from build123d import *

# Parameters (mm, degrees)
SKETCH1_R           = 2
BOSS_EXTRUDE1_DEPTH = 3


with BuildPart() as part:
    # Sketch1 → Boss-Extrude1 (new body)
    with BuildSketch(Plane(origin=(0, 0, 0), x_dir=(1, 0, 0), z_dir=(0, 1, 0))):
        Polygon((-117.708234781, 46.18565323), (-117.708234781, 37.539058804), (-104.708234781, 37.539058804), (-104.708234781, -32.460941196), (-117.708234781, -32.460941196), (-117.708234781, -41.961747622), (-102.708234781, -57.460941196), (-32.708234781, -57.460941196), (-17.708234781, -41.961747622), (-17.708234781, -32.460941196), (-30.708234781, -32.460941196), (-30.708234781, 37.539058804), (-17.708234781, 37.539058804), (-17.708234781, 48.362937983), (-32.482765457, 62.539058804), (-102.482765457, 62.539058804), (-117.673238758, 46.131294908), align=None)
        with Locations((-96.708234781, 16.539058804)):
            Circle(SKETCH1_R, mode=Mode.SUBTRACT)
        with Locations((-96.708234781, -11.460941196)):
            Circle(SKETCH1_R, mode=Mode.SUBTRACT)
        with Locations((-102.708234781, -48.800687158)):
            Circle(SKETCH1_R, mode=Mode.SUBTRACT)
        with Locations((-67.708234781, -48.800687158)):
            Circle(SKETCH1_R, mode=Mode.SUBTRACT)
        with Locations((-102.708234781, 53.878804766)):
            Circle(SKETCH1_R, mode=Mode.SUBTRACT)
        with Locations((-67.708234781, 53.878804766)):
            Circle(SKETCH1_R, mode=Mode.SUBTRACT)
        with Locations((-32.708234781, 53.878804766)):
            Circle(SKETCH1_R, mode=Mode.SUBTRACT)
        with Locations((-32.708234781, -48.800687158)):
            Circle(SKETCH1_R, mode=Mode.SUBTRACT)
        with Locations((-38.708234781, -11.460941196)):
            Circle(SKETCH1_R, mode=Mode.SUBTRACT)
        with Locations((-38.708234781, 16.539058804)):
            Circle(SKETCH1_R, mode=Mode.SUBTRACT)
        with Locations((-52.771353365, 2.539058804)):
            Circle(SKETCH1_R, mode=Mode.SUBTRACT)
        with Locations((-82.645116197, 2.539058804)):
            Circle(SKETCH1_R, mode=Mode.SUBTRACT)
        with BuildLine():
            Line((-79.583025643, 48.362937983), (-79.583025643, 23.355939616))
            ThreePointArc((-79.583025643, 23.355939616), (-81.595082983, 21.343882276), (-83.607140323, 23.355939616))
            Line((-83.607140323, 23.355939616), (-83.607140323, 48.362937983))
            ThreePointArc((-83.607140323, 48.362937983), (-81.595082983, 50.374995323), (-79.583025643, 48.362937983))
        make_face(mode=Mode.SUBTRACT)
        with BuildLine():
            Line((-71.954133984, 48.07550122), (-71.954133984, 23.068502853))
            ThreePointArc((-71.954133984, 23.068502853), (-73.966191324, 21.056445514), (-75.978248664, 23.068502853))
            Line((-75.978248664, 23.068502853), (-75.978248664, 48.07550122))
            ThreePointArc((-75.978248664, 48.07550122), (-73.966191324, 50.08755856), (-71.954133984, 48.07550122))
        make_face(mode=Mode.SUBTRACT)
        with BuildLine():
            Line((-73.966191324, 14.281397024), (-91.218060864, 14.281397024))
            ThreePointArc((-91.218060864, 14.281397024), (-93.048616644, 16.111952804), (-91.218060864, 17.942508584))
            Line((-91.218060864, 17.942508584), (-73.966191324, 17.942508584))
            ThreePointArc((-73.966191324, 17.942508584), (-72.135635543, 16.111952804), (-73.966191324, 14.281397024))
        make_face(mode=Mode.SUBTRACT)
        with BuildLine():
            Line((-96.834895183, 48.362937983), (-96.834895183, 23.355939616))
            ThreePointArc((-96.834895183, 23.355939616), (-98.846952522, 21.343882276), (-100.859009862, 23.355939616))
            Line((-100.859009862, 23.355939616), (-100.859009862, 48.362937983))
            ThreePointArc((-100.859009862, 48.362937983), (-98.846952522, 50.374995323), (-96.834895183, 48.362937983))
        make_face(mode=Mode.SUBTRACT)
        with BuildLine():
            Line((-89.206003524, 48.07550122), (-89.206003524, 23.068502853))
            ThreePointArc((-89.206003524, 23.068502853), (-91.218060864, 21.056445514), (-93.230118203, 23.068502853))
            Line((-93.230118203, 23.068502853), (-93.230118203, 48.07550122))
            ThreePointArc((-93.230118203, 48.07550122), (-91.218060864, 50.08755856), (-89.206003524, 48.07550122))
        make_face(mode=Mode.SUBTRACT)
        with BuildLine():
            Line((-55.727463713, 48.362937983), (-55.727463713, 23.355939616))
            ThreePointArc((-55.727463713, 23.355939616), (-53.715406373, 21.343882276), (-51.703349033, 23.355939616))
            Line((-51.703349033, 23.355939616), (-51.703349033, 48.362937983))
            ThreePointArc((-51.703349033, 48.362937983), (-53.715406373, 50.374995323), (-55.727463713, 48.362937983))
        make_face(mode=Mode.SUBTRACT)
        with BuildLine():
            Line((-63.356355372, 48.07550122), (-63.356355372, 23.068502853))
            ThreePointArc((-63.356355372, 23.068502853), (-61.344298032, 21.056445514), (-59.332240692, 23.068502853))
            Line((-59.332240692, 23.068502853), (-59.332240692, 48.07550122))
            ThreePointArc((-59.332240692, 48.07550122), (-61.344298032, 50.08755856), (-63.356355372, 48.07550122))
        make_face(mode=Mode.SUBTRACT)
        with BuildLine():
            Line((-38.475594173, 48.362937983), (-38.475594173, 23.355939616))
            ThreePointArc((-38.475594173, 23.355939616), (-36.463536833, 21.343882276), (-34.451479493, 23.355939616))
            Line((-34.451479493, 23.355939616), (-34.451479493, 48.362937983))
            ThreePointArc((-34.451479493, 48.362937983), (-36.463536833, 50.374995323), (-38.475594173, 48.362937983))
        make_face(mode=Mode.SUBTRACT)
        with BuildLine():
            Line((-46.104485832, 48.07550122), (-46.104485832, 23.068502853))
            ThreePointArc((-46.104485832, 23.068502853), (-44.092428492, 21.056445514), (-42.080371152, 23.068502853))
            Line((-42.080371152, 23.068502853), (-42.080371152, 48.07550122))
            ThreePointArc((-42.080371152, 48.07550122), (-44.092428492, 50.08755856), (-46.104485832, 48.07550122))
        make_face(mode=Mode.SUBTRACT)
        with BuildLine():
            Line((-79.583025643, -44.139032376), (-79.583025643, -19.132034009))
            ThreePointArc((-79.583025643, -19.132034009), (-81.595082983, -17.119976669), (-83.607140323, -19.132034009))
            Line((-83.607140323, -19.132034009), (-83.607140323, -44.139032376))
            ThreePointArc((-83.607140323, -44.139032376), (-81.595082983, -46.151089715), (-79.583025643, -44.139032376))
        make_face(mode=Mode.SUBTRACT)
        with BuildLine():
            Line((-71.954133984, -43.851595613), (-71.954133984, -18.844597246))
            ThreePointArc((-71.954133984, -18.844597246), (-73.966191324, -16.832539906), (-75.978248664, -18.844597246))
            Line((-75.978248664, -18.844597246), (-75.978248664, -43.851595613))
            ThreePointArc((-75.978248664, -43.851595613), (-73.966191324, -45.863652953), (-71.954133984, -43.851595613))
        make_face(mode=Mode.SUBTRACT)
        with BuildLine():
            Line((-96.834895183, -44.139032376), (-96.834895183, -19.132034009))
            ThreePointArc((-96.834895183, -19.132034009), (-98.846952522, -17.119976669), (-100.859009862, -19.132034009))
            Line((-100.859009862, -19.132034009), (-100.859009862, -44.139032376))
            ThreePointArc((-100.859009862, -44.139032376), (-98.846952522, -46.151089715), (-96.834895183, -44.139032376))
        make_face(mode=Mode.SUBTRACT)
        with BuildLine():
            Line((-89.206003524, -43.851595613), (-89.206003524, -18.844597246))
            ThreePointArc((-89.206003524, -18.844597246), (-91.218060864, -16.832539906), (-93.230118203, -18.844597246))
            Line((-93.230118203, -18.844597246), (-93.230118203, -43.851595613))
            ThreePointArc((-93.230118203, -43.851595613), (-91.218060864, -45.863652953), (-89.206003524, -43.851595613))
        make_face(mode=Mode.SUBTRACT)
        with BuildLine():
            Line((-55.727463713, -44.139032376), (-55.727463713, -19.132034009))
            ThreePointArc((-55.727463713, -19.132034009), (-53.715406373, -17.119976669), (-51.703349033, -19.132034009))
            Line((-51.703349033, -19.132034009), (-51.703349033, -44.139032376))
            ThreePointArc((-51.703349033, -44.139032376), (-53.715406373, -46.151089715), (-55.727463713, -44.139032376))
        make_face(mode=Mode.SUBTRACT)
        with BuildLine():
            Line((-63.356355372, -43.851595613), (-63.356355372, -18.844597246))
            ThreePointArc((-63.356355372, -18.844597246), (-61.344298032, -16.832539906), (-59.332240692, -18.844597246))
            Line((-59.332240692, -18.844597246), (-59.332240692, -43.851595613))
            ThreePointArc((-59.332240692, -43.851595613), (-61.344298032, -45.863652953), (-63.356355372, -43.851595613))
        make_face(mode=Mode.SUBTRACT)
        with BuildLine():
            Line((-38.475594173, -44.139032376), (-38.475594173, -19.132034009))
            ThreePointArc((-38.475594173, -19.132034009), (-36.463536833, -17.119976669), (-34.451479493, -19.132034009))
            Line((-34.451479493, -19.132034009), (-34.451479493, -44.139032376))
            ThreePointArc((-34.451479493, -44.139032376), (-36.463536833, -46.151089715), (-38.475594173, -44.139032376))
        make_face(mode=Mode.SUBTRACT)
        with BuildLine():
            Line((-46.104485832, -43.851595613), (-46.104485832, -18.844597246))
            ThreePointArc((-46.104485832, -18.844597246), (-44.092428492, -16.832539906), (-42.080371152, -18.844597246))
            Line((-42.080371152, -18.844597246), (-42.080371152, -43.851595613))
            ThreePointArc((-42.080371152, -43.851595613), (-44.092428492, -45.863652953), (-46.104485832, -43.851595613))
        make_face(mode=Mode.SUBTRACT)
        with BuildLine():
            Line((-73.966191324, 7.984384289), (-91.218060864, 7.984384289))
            ThreePointArc((-91.218060864, 7.984384289), (-92.918765354, 9.685088779), (-91.218060864, 11.385793269))
            Line((-91.218060864, 11.385793269), (-73.966191324, 11.385793269))
            ThreePointArc((-73.966191324, 11.385793269), (-72.265486834, 9.685088779), (-73.966191324, 7.984384289))
        make_face(mode=Mode.SUBTRACT)
        with BuildLine():
            Line((-61.344298032, 14.281397024), (-44.092428492, 14.281397024))
            ThreePointArc((-44.092428492, 14.281397024), (-42.261872712, 16.111952804), (-44.092428492, 17.942508584))
            Line((-44.092428492, 17.942508584), (-61.344298032, 17.942508584))
            ThreePointArc((-61.344298032, 17.942508584), (-63.174853812, 16.111952804), (-61.344298032, 14.281397024))
        make_face(mode=Mode.SUBTRACT)
        with BuildLine():
            Line((-61.344298032, 7.984384289), (-44.092428492, 7.984384289))
            ThreePointArc((-44.092428492, 7.984384289), (-42.391724002, 9.685088779), (-44.092428492, 11.385793269))
            Line((-44.092428492, 11.385793269), (-61.344298032, 11.385793269))
            ThreePointArc((-61.344298032, 11.385793269), (-63.045002522, 9.685088779), (-61.344298032, 7.984384289))
        make_face(mode=Mode.SUBTRACT)
        with BuildLine():
            Line((-73.966191324, -10.057491416), (-91.218060864, -10.057491416))
            ThreePointArc((-91.218060864, -10.057491416), (-93.048616644, -11.888047196), (-91.218060864, -13.718602976))
            Line((-91.218060864, -13.718602976), (-73.966191324, -13.718602976))
            ThreePointArc((-73.966191324, -13.718602976), (-72.135635543, -11.888047196), (-73.966191324, -10.057491416))
        make_face(mode=Mode.SUBTRACT)
        with BuildLine():
            Line((-73.966191324, -3.760478681), (-91.218060864, -3.760478681))
            ThreePointArc((-91.218060864, -3.760478681), (-92.918765354, -5.461183171), (-91.218060864, -7.161887662))
            Line((-91.218060864, -7.161887662), (-73.966191324, -7.161887662))
            ThreePointArc((-73.966191324, -7.161887662), (-72.265486834, -5.461183171), (-73.966191324, -3.760478681))
        make_face(mode=Mode.SUBTRACT)
        with BuildLine():
            Line((-61.344298032, -10.057491416), (-44.092428492, -10.057491416))
            ThreePointArc((-44.092428492, -10.057491416), (-42.261872712, -11.888047196), (-44.092428492, -13.718602976))
            Line((-44.092428492, -13.718602976), (-61.344298032, -13.718602976))
            ThreePointArc((-61.344298032, -13.718602976), (-63.174853812, -11.888047196), (-61.344298032, -10.057491416))
        make_face(mode=Mode.SUBTRACT)
        with BuildLine():
            Line((-61.344298032, -3.760478681), (-44.092428492, -3.760478681))
            ThreePointArc((-44.092428492, -3.760478681), (-42.391724002, -5.461183171), (-44.092428492, -7.161887662))
            Line((-44.092428492, -7.161887662), (-61.344298032, -7.161887662))
            ThreePointArc((-61.344298032, -7.161887662), (-63.045002522, -5.461183171), (-61.344298032, -3.760478681))
        make_face(mode=Mode.SUBTRACT)
    extrude(amount=BOSS_EXTRUDE1_DEPTH)


solid = part.part
Design review of the part built by this model. Coordinates are the model's own, in mm. Round coordinates to 2 decimals unless told otherwise and drop trailing zeros. Write each loop counter-clockwise with the first axis right and the second up, starting at its lowest first coordinate (ties: lowest second). Pieces come first, ordered by that corner, then holes. Notation, with made-up numbers: (-22.5, 79) -> (-8.5, 79) arc R26 cw to (-8.5, 118) -> close; hole circle Ø10 at (24.5, -19.75). An arc over 180 degrees is marked (long way). One line per item, written item: value. Start each with the question number.
Q1. To check wall thickness, follow probe 1 along Z at (x, y) = (-86.5, 0.4); probe 2 along X at (y, z) = (1.7, 47); probe 3 along Z at (x, y) = (-99, 1.1). State the ranges of each line that lie inside material, in increasing order.
Q2. The part is to be moulded in two halves that separate along X. For faces 1 (the face through (-36.8, 1.48, -17.14)), 2 (the face through (-111, 1, -37.539)), say which applies: pulls with the +X half, pulls with the -X half, needs draft (parallel to the pull), parting line crosses it, or undercut.
Q3. Add section B-B (z = -32). State how many separate pieces and enclosed holes the cut face has, then the cut area to 3 significant figures.
Q4. Add section A-A (x = -28.5). Give the boundary of the cut face in (y, z).
Q5. Insertion check: P1, Ø2, axis at x = -48.5, z = -34.5, coming from the -Y side; P2, Ø1.5, axis at y = 1.5, z = -33, coming from the -X side; P3, Ø1.5, axis at y = 1, z = -31, coming from the +X side. Each pin has a flat end and moves straight along its axis. Give the tip position at first contact, or say it passes through.
Response:
1. probe 1: z = -62.54 to -17.94, -14.28 to -11.39, -7.98 to 3.76, 7.16 to 10.06, 13.72 to 57.46
1. probe 2: x = -112.83 to -103.58, -101.84 to -68.58, -66.84 to -33.58, -31.84 to -22.58
1. probe 3: z = -62.54 to -50.37, -21.35 to 17.13, 46.15 to 57.46
2. face 1: undercut
2. face 2: needs draft
3. separate pieces: 9
3. enclosed holes: 0
3. area: 125 mm^2
4. outline: (0, -58.72) -> (3, -58.72) -> (3, -37.54) -> (0, -37.54) -> close; (0, 32.46) -> (3, 32.46) -> (3, 53.11) -> (0, 53.11) -> close
5. P1: stops at y = 0
5. P2: stops at x = -104.71
5. P3: stops at x = -30.71
